Source: CAD feature listing. Evaluate the final solid. Frame: model axes, mm. Face numbers are marked on the shaded views. A direction names the side the tool comes from. Coordinates: 2 decimals unless noted, no trailing zeros. Order: outer loops, then holes, each group sorted by start corner. A loop starts at its lowest first (then second) coordinate and runs counter-clockwise, first axis right, second up. Notation, with made-up numbers: (23.25, 79) -> (40.25, 79) arc R30 cw to (40.25, 110) -> close; hole circle Ø2 at (17, 36). An arc over 180 degrees is marked (long way). Write each question's results on one line, items separated by ' | '. Start each with the question number.
from build123d import *

# Parameters (mm, degrees)
BOSS_EXTRUDE1_DEPTH = 15.875
SKETCH2_W           = 15.875
SKETCH2_H           = 6.35
BOSS_EXTRUDE2_DEPTH = 6.35
BOSS_EXTRUDE3_DEPTH = 6.35
SKETCH4_W           = 6.35
SKETCH4_H           = 1.27
CUT_EXTRUDE1_DEPTH  = 6.35


with BuildPart() as part:
    # Sketch1 → Boss-Extrude1 (new body)
    with BuildSketch(Plane.XY):
        Polygon((0, 0), (0, 25.4), (3.175, 25.4), (25.4, 3.175), (25.4, 0), align=None)
    extrude(amount=BOSS_EXTRUDE1_DEPTH)

    # Sketch2 → Boss-Extrude2 (add)
    with BuildSketch(Plane.ZY):
        with Locations((7.9375, 15.24)):
            Rectangle(SKETCH2_W, SKETCH2_H)
    boss_extrude2 = extrude(amount=BOSS_EXTRUDE2_DEPTH)

    # Sketch3 → Boss-Extrude3 (add)
    with BuildSketch(Plane(origin=(0, 18.415, 0), x_dir=(1, 0, 0), z_dir=(0, 1, 0))):
        Polygon((-9.35, -14.907), (-9.35, -13.875), (-6.35, -13.875), (-6.35, -15.875), (-6.858, -16.383), (-7.874, -16.383), align=None)
        Polygon((-7.874, 0.508), (-9.35, -0.968), (-9.35, -2), (-6.35, -2), (-6.35, 0), (-6.858, 0.508), align=None)
    boss_extrude3 = extrude(amount=-BOSS_EXTRUDE3_DEPTH)

    # Sketch4 → Cut-Extrude1 (cut)
    with BuildSketch(Plane(origin=(0, 18.415, 0), x_dir=(1, 0, 0), z_dir=(0, 1, 0))):
        with Locations((-3.175, -13.24)):
            Rectangle(SKETCH4_W, SKETCH4_H)
        with Locations((-3.175, -2.635)):
            Rectangle(SKETCH4_W, SKETCH4_H)
    cut_extrude1 = extrude(amount=-CUT_EXTRUDE1_DEPTH, mode=Mode.SUBTRACT)

    # Mirror1: Boss-Extrude2, Boss-Extrude3, Cut-Extrude1 across plane
    add(boss_extrude2.mirror(Plane(origin=(0, 0, 0), x_dir=(0, 0, 1), z_dir=(0.7071067811865476, -0.7071067811865476, 0))))
    add(boss_extrude3.mirror(Plane(origin=(0, 0, 0), x_dir=(0, 0, 1), z_dir=(0.7071067811865476, -0.7071067811865476, 0))))
    add(cut_extrude1.mirror(Plane(origin=(0, 0, 0), x_dir=(0, 0, 1), z_dir=(0.7071067811865476, -0.7071067811865476, 0))), mode=Mode.SUBTRACT)


solid = part.part
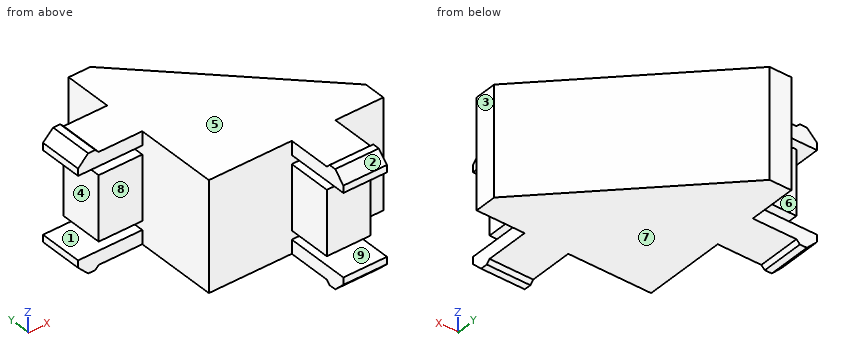
(1) Section A-A on x = -1. Return the cut outline in (y, z) (3 decimals), then the cut area to 3 significant figures.
(2) Section D-D on x = 14.5. Return the cut outline in (y, z) (3 decimals).
(3) Section B-B on z = 1.5. Return the cut outline in (x, y) (3 decimals).
(4) Line query: L1, parallel to Z at x = 14, y = -5.5 (3 decimals); L2, parallel to Y at x = 2, z = 15.5; L3, parallel to X at y = -6, z = 15 (3 decimals). Output: solid intervals per line, ascending.
(5) Draft query along Z for the marked faces 1, 2, 3 and 4. Return one class per face: released by +Z, released by -Z, zero draft, split by the parting line, or undercut.
(6) Reachability of the marked faces 5, 6, 7, 8 and 9 from +Z, -Z, +X, -X, +Y, -Y: full face, straight path, thin tool, end or side. Return the list, or none.
(7) Section C-C on y = 16.5. Return the cut outline in (x, z) (3 decimals).
(8) First-contact query: P1, Ø5, axis at x = 13.5, y = 8.5, coming from the +Z side (3 decimals); P2, Ø3, axis at y = 19.5, z = 10, coming from the +X side (3 decimals); P3, Ø1.3, axis at y = -3, z = 15, coming from the -X side (3 decimals). Flat tips, straight axial feed; report the tip coordinate or a pass-through.
Results list:
1) outline: (12.065, 0) -> (18.415, 0) -> (18.415, 2) -> (12.065, 2) -> close; (12.065, 3.27) -> (18.415, 3.27) -> (18.415, 12.605) -> (12.065, 12.605) -> close; (12.065, 13.875) -> (18.415, 13.875) -> (18.415, 15.875) -> (12.065, 15.875) -> close | area: 84.7 mm²
2) outline: (-9.35, 0.968) -> (-7.874, -0.508) -> (-6.858, -0.508) -> (-6.35, 0) -> (14.075, 0) -> (14.075, 15.875) -> (-6.35, 15.875) -> (-6.858, 16.383) -> (-7.874, 16.383) -> (-9.35, 14.907) -> (-9.35, 13.875) -> (0, 13.875) -> (0, 12.605) -> (-6.35, 12.605) -> (-6.35, 3.27) -> (0, 3.27) -> (0, 2) -> (-9.35, 2) -> close
3) outline: (-9.35, 12.065) -> (0, 12.065) -> (0, 0) -> (12.065, 0) -> (12.065, -9.35) -> (18.415, -9.35) -> (18.415, 0) -> (25.4, 0) -> (25.4, 3.175) -> (3.175, 25.4) -> (0, 25.4) -> (0, 18.415) -> (-9.35, 18.415) -> close
4) L1: z = 0 to 2, 3.27 to 12.605, 13.875 to 15.875 | L2: y = 0 to 25.4 | L3: x = 12.065 to 18.415
5) face 1: undercut | face 2: released by +Z | face 3: zero draft | face 4: undercut
6) face 5: +Z, +X, +Y | face 6: +Z, -Z, -X, +Y | face 7: -Z, +X, +Y | face 8: +Z, -Z, -X, -Y | face 9: +X, -X, -Y
7) outline: (-9.35, 0.968) -> (-7.874, -0.508) -> (-6.858, -0.508) -> (-6.35, 0) -> (12.075, 0) -> (12.075, 15.875) -> (-6.35, 15.875) -> (-6.858, 16.383) -> (-7.874, 16.383) -> (-9.35, 14.907) -> (-9.35, 13.875) -> (0, 13.875) -> (0, 12.605) -> (-6.35, 12.605) -> (-6.35, 3.27) -> (0, 3.27) -> (0, 2) -> (-9.35, 2) -> close
8) P1: stops at z = 15.875 | P2: stops at x = 10.575 | P3: stops at x = 12.065
